```python
from build123d import *

# Parameters (mm, degrees)
BOX005_W               = 11
BOX005_H               = 20
BOX005_DEPTH           = 8
CYLINDER002_R          = 1.6
CYLINDER002_DEPTH      = 19
CYLINDER002_ROLL_ANGLE = 90
BOX001_W               = 15
BOX001_H               = 11
BOX001_DEPTH           = 7
BOX_W                  = 11
BOX_H                  = 19
BOX_DEPTH              = 8
CHAMFER_SIZE           = 3
CHAMFER001_SIZE        = 3
CHAMFER003_SIZE        = 3
CHAMFER004_SIZE        = 3
CYLINDER005_R          = 3
CYLINDER005_DEPTH      = 19
CYLINDER005_ROLL_ANGLE = 90
CYLINDER007_R          = 1.5
CYLINDER007_DEPTH      = 6
CYLINDER007_ROLL_ANGLE = 90
BOX004_W               = 10
BOX004_H               = 6
BOX004_DEPTH           = 4
CYLINDER008_R          = 3
CYLINDER008_DEPTH      = 6
CYLINDER008_ROLL_ANGLE = 90
CYLINDER003_R          = 1.5
CYLINDER003_DEPTH      = 6
CYLINDER003_ROLL_ANGLE = 90
BOX002_W               = 10
BOX002_H               = 6
BOX002_DEPTH           = 4
CYLINDER004_R          = 3
CYLINDER004_DEPTH      = 6
CYLINDER004_ROLL_ANGLE = 90


with BuildPart() as cube005:
    # Box005 → Box005 (new body)
    with BuildSketch(Plane(origin=(11, -0.5, 0), x_dir=(1, 0, 0), z_dir=(0, 0, 1))):
        with Locations((5.5, 10)):
            Rectangle(BOX005_W, BOX005_H)
    extrude(amount=BOX005_DEPTH)


with BuildPart() as cylinder001:
    # Cylinder002 → Cylinder002 (new body)
    with BuildSketch(Plane.XY):
        Circle(CYLINDER002_R)
    extrude(amount=CYLINDER002_DEPTH)


with BuildPart() as cylinder001_1:
    # Cylinder002 roll: moved
    add(cylinder001.part.rotate(Axis((0, 0, 0), (1, 0, 0)), CYLINDER002_ROLL_ANGLE))


with BuildPart() as cylinder001_2:
    # Cylinder002 placement: moved
    add(cylinder001_1.part.moved(Location((-0.5, 19, 4.5))))


with BuildPart() as cube001:
    # Box001 → Box001 (new body)
    with BuildSketch(Plane(origin=(0, 4, 2), x_dir=(1, 0, 0), z_dir=(0, 0, 1))):
        with Locations((7.5, 5.5)):
            Rectangle(BOX001_W, BOX001_H)
    extrude(amount=BOX001_DEPTH)


with BuildPart() as chamfer004:
    # Box → Box (new body)
    with BuildSketch(Plane.XY):
        with Locations((5.5, 9.5)):
            Rectangle(BOX_W, BOX_H)
    extrude(amount=BOX_DEPTH)

    # Chamfer
    chamfer_edges = [chamfer004.edges().sort_by_distance(p)[0] for p in [
        (11, 9.5, 8),
    ]]
    chamfer(chamfer_edges, length=CHAMFER_SIZE)

    # Chamfer001
    chamfer001_edges = [chamfer004.edges().sort_by_distance(p)[0] for p in [
        (0, 9.5, 8),
    ]]
    chamfer(chamfer001_edges, length=CHAMFER001_SIZE)

    # Cut003: cut Cube001
    add(cube001.part, mode=Mode.SUBTRACT)

    # Chamfer003
    chamfer003_edges = [chamfer004.edges().sort_by_distance(p)[0] for p in [
        (5.5, 15, 8),
    ]]
    chamfer(chamfer003_edges, length=CHAMFER003_SIZE)

    # Chamfer004
    chamfer004_edges = [chamfer004.edges().sort_by_distance(p)[0] for p in [
        (5.5, 4, 8),
    ]]
    chamfer(chamfer004_edges, length=CHAMFER004_SIZE)


with BuildPart() as obj1:
    # Cylinder005 → Cylinder005 (new body)
    with BuildSketch(Plane.XY):
        Circle(CYLINDER005_R)
    extrude(amount=CYLINDER005_DEPTH)


with BuildPart() as obj1_1:
    # Cylinder005 roll: moved
    add(obj1.part.rotate(Axis((0, 0, 0), (1, 0, 0)), CYLINDER005_ROLL_ANGLE))


with BuildPart() as obj1_2:
    # Cylinder005 placement: moved
    add(obj1_1.part.moved(Location((-0.5, 19, 4.5))))

    # Fusion001: union Chamfer004
    add(chamfer004.part)

    # Cut004: cut Cylinder001
    add(cylinder001_2.part, mode=Mode.SUBTRACT)


with BuildPart() as cylinder029:
    # Cylinder007 → Cylinder007 (new body)
    with BuildSketch(Plane.XY):
        Circle(CYLINDER007_R)
    extrude(amount=CYLINDER007_DEPTH)


with BuildPart() as cylinder029_1:
    # Cylinder007 roll: moved
    add(cylinder029.part.rotate(Axis((0, 0, 0), (1, 0, 0)), CYLINDER007_ROLL_ANGLE))


with BuildPart() as cylinder029_2:
    # Cylinder007 placement: moved
    add(cylinder029_1.part.moved(Location((15.5, 25, 4.5))))


with BuildPart() as cube004:
    # Box004 → Box004 (new body)
    with BuildSketch(Plane(origin=(5, 19, 0), x_dir=(1, 0, 0), z_dir=(0, 0, 1))):
        with Locations((5, 3)):
            Rectangle(BOX004_W, BOX004_H)
    extrude(amount=BOX004_DEPTH)


with BuildPart() as obj2:
    # Cylinder008 → Cylinder008 (new body)
    with BuildSketch(Plane.XY):
        Circle(CYLINDER008_R)
    extrude(amount=CYLINDER008_DEPTH)


with BuildPart() as obj2_1:
    # Cylinder008 roll: moved
    add(obj2.part.rotate(Axis((0, 0, 0), (1, 0, 0)), CYLINDER008_ROLL_ANGLE))


with BuildPart() as obj2_2:
    # Cylinder008 placement: moved
    add(obj2_1.part.moved(Location((15, 25, 4.5))))

    # Fusion002: union Cube004
    add(cube004.part)


with BuildPart() as obj2_3:
    # Fusion002 placement: moved
    add(obj2_2.part.moved(Location((0.5, 0, 0))))

    # Cut005: cut Cylinder029
    add(cylinder029_2.part, mode=Mode.SUBTRACT)


with BuildPart() as cylinder002:
    # Cylinder003 → Cylinder003 (new body)
    with BuildSketch(Plane.XY):
        Circle(CYLINDER003_R)
    extrude(amount=CYLINDER003_DEPTH)


with BuildPart() as cylinder002_1:
    # Cylinder003 roll: moved
    add(cylinder002.part.rotate(Axis((0, 0, 0), (1, 0, 0)), CYLINDER003_ROLL_ANGLE))


with BuildPart() as cylinder002_2:
    # Cylinder003 placement: moved
    add(cylinder002_1.part.moved(Location((15.5, 0, 4.5))))


with BuildPart() as cube002:
    # Box002 → Box002 (new body)
    with BuildSketch(Plane(origin=(5, -6, 0), x_dir=(1, 0, 0), z_dir=(0, 0, 1))):
        with Locations((5, 3)):
            Rectangle(BOX002_W, BOX002_H)
    extrude(amount=BOX002_DEPTH)


with BuildPart() as obj3:
    # Cylinder004 → Cylinder004 (new body)
    with BuildSketch(Plane.XY):
        Circle(CYLINDER004_R)
    extrude(amount=CYLINDER004_DEPTH)


with BuildPart() as obj3_1:
    # Cylinder004 roll: moved
    add(obj3.part.rotate(Axis((0, 0, 0), (1, 0, 0)), CYLINDER004_ROLL_ANGLE))


with BuildPart() as obj3_2:
    # Cylinder004 placement: moved
    add(obj3_1.part.moved(Location((15, 0, 4.5))))

    # Fusion: union Cube002
    add(cube002.part)


with BuildPart() as obj3_3:
    # Fusion placement: moved
    add(obj3_2.part.moved(Location((0.5, 0, 0))))

    # Cut002: cut Cylinder002
    add(cylinder002_2.part, mode=Mode.SUBTRACT)

    # Fusion003: union obj1, obj2
    add(obj1_2.part)
    add(obj2_3.part)

    # Cut006: cut Cube005
    add(cube005.part, mode=Mode.SUBTRACT)


solid = obj3_3.part
```
The listing builds one solid part. Answer for the finished solid, in the listing's coordinates (mm). A direction names the side the tool comes from. Coordinates: 2 decimals unless noted, no trailing zeros. Write each loop counter-clockwise with the first axis right and the second up, starting at its lowest first coordinate (ties: lowest second). Pieces come first, ordered by that corner, then holes. Notation, with made-up numbers: (71.5, 3) - (102.5, 3) arc R10 ccw to (102.5, 13) - close; hole circle Ø4 at (-40, -13). An arc over 180 degrees is marked (long way). Return JSON: item names as keys, results as strings. Group by question number.
Q1. The part is cut by section B-B on y = 2. Write down the section's boundary in (x, z), and give its area (3 significant figures).
Q2. Flat-ended cylindrical pins translate along their axes: pin 1 Ø3.5 at (x, z) = (-0.5, 4.5) entering from -Y; pin 2 Ø1.5 at (y, z) = (6, 3.5) entering from -X; pin 3 Ø0.8 at (y, z) = (13.5, 1) entering from -X; pin 4 Ø3.5 at (x, z) = (15.5, 4.5) entering from -Y. Find the tip coordinate at first contact, or state that the pin passes through.
Q3. Which of the six approach directions +Z, -Z, +X, -X, +Y, -Y give full straight-line access (tool end or side, diameter ignored) to faces 4 (the flat face through (2, 1, 7)), 5 (the flat face through (5.5, -3, 2)), 6 (the flat face through (5, 17, 7))?
Q4. The part is cut by section A-A on x = -0.5. Write down the section's boundary in (y, z).
Q5. The part is cut by section D-D on x = 12. Write down the section's boundary in (y, z), and give its area (3 significant figures).
Q6. Find the intervals of material crossed by line 1 along Y through (x, z) = (8.75, 4.5); line 2 along Z through (x, y) = (-0.5, 13.5); line 3 along X through (y, z) = (22.7, 4.5), in increasing order. Write a range as [from, to].
Q7. The part is cut by section C-C on z = 5.5. Write down the section's boundary in (x, y).
Q8. For a pull along Y with two mould halves and no side action, classify faces 1 (the flat face through (5, 2, 7)), 2 (the flat face through (12, 25, 3)), 3 (the flat face through (15.5, 22, 1)) as +Y half, -Y half, draft (parallel to the pull), parting line (faces both ways), or undercut.
Evaluation:
{
 "1": {"outline": "(0, 0) - (11, 0) - (11, 5) - (9, 7) - (2, 7) - (1.62, 6.62) arc R3 ccw (long way) to (0, 1.54) - close; hole circle Ø3.2 at (-0.5, 4.5)", "area": "84.2 mm2"},
 "2": {"pin 1": "stops at y = 0", "pin 2": "stops at x = -3.49", "pin 3": "stops at x = 0", "pin 4": "stops at y = -6"},
 "3": {"face 4": "+Z, +Y, -Y", "face 5": "+Z, -Z, -X, -Y", "face 6": "+Z, +X"},
 "4": {"outline": "(0, 1.5) - (19, 1.5) - (19, 2.9) - (0, 2.9) - close; (0, 6.1) - (19, 6.1) - (19, 7.5) - (0, 7.5) - close"},
 "5": {"outline": "(-6, 0) - (-0.5, 0) - (-0.5, 4) - (-6, 4) - close; (19.5, 0) - (25, 0) - (25, 4) - (19.5, 4) - close", "area": "44.0 mm2"},
 "6": {"line 1": "y = [0, 4], [15, 19]", "line 2": "z = [1.5, 2.9], [6.1, 7.5]", "line 3": "x = [12.5, 14], [17, 18.5]"},
 "7": {"outline": "(-3.33, 0) - (-1.75, 0) - (-1.75, 19) - (-3.33, 19) - close; (0.75, 0) - (10.5, 0) - (10.5, 3.5) - (2.33, 3.5) - (2.33, 15.5) - (10.5, 15.5) - (10.5, 19) - (0.75, 19) - close; (12.67, -6) - (14.38, -6) - (14.38, -0.5) - (12.67, -0.5) - close; (12.67, 19.5) - (14.38, 19.5) - (14.38, 25) - (12.67, 25) - close; (16.62, -6) - (18.33, -6) - (18.33, -0.5) - (16.62, -0.5) - close; (16.62, 19.5) - (18.33, 19.5) - (18.33, 25) - (16.62, 25) - close"},
 "8": {"face 1": "undercut", "face 2": "+Y half", "face 3": "draft"}
}
